CAD build for the part. Positions are in the model's coordinates, mm. A direction names the side the tool comes from. Give positions to 0.01 mm unless a question says otherwise; leave off trailing zeros. Write each loop counter-clockwise with the first axis right and the second up, starting at its lowest first coordinate (ties: lowest second). Pieces come first, ordered by that corner, then holes. Notation, with made-up numbers: (13.25, -35.5) - (22.25, -35.5) arc R18 cw to (22.25, -26.5) - close; hole circle Ø6 at (58.25, 39). An arc over 180 degrees is marked (long way). Put each result on its own line as item: value. Start each with the question number.
1. Tool access for faces 1 (the flat face through (-3, -47.498, 12.2)), 2 (the flat face through (0, -60.198, 7)): list every direction of +Z, -Z, +X, -X, +Y, -Y with a clear straight run to the whole face (end or side of a thin tool).
2. Cut at C-C on y = -6. List the corners of the cut face in (x, z).
3. Cut at D-D on y = -49.5. List the corners of the cut face in (x, z), and give its area (3 significant figures).
4. Cut at B-B on z = 6.35. List the corners of the cut face in (x, y).
5. Wall check: line 1 (X direction, y = -53, z = 7); line 2 (Y direction, x = -1.25, z = -0.75); line 3 (Z direction, x = 0.25, y = -42). Give the ranges that are in metal, low to high.
6. Cut at A-A on x = 0. List the corners of the cut face in (y, z).
7. Drop flat-ended pins along their axis: pin 1 (2 mm diameter, centred on x = 9, y = -8.5, fed in from +Z); pin 2 (3 mm diameter, centred on x = -6.5, y = 35.5, fed in from -Z); pin 3 (12 mm diameter, centred on x = 8, y = -43, fed in from +Z); pin 4 (12 mm diameter, centred on y = -32.5, z = 0, fed in from -X). Give the stop position or say it passes through.
from build123d import *

# Parameters (mm, degrees)
F0_R       = 6.35
F1_DEPTH   = 101.6
F1_FACE1_R = 6.35
F2_R       = 12.7
F2_R_2     = 6.35
F1_FACE_R  = 6.35
F3_DEPTH   = 6.35


with BuildPart() as f1:
    # F0 (on Front) → F1 (new body)
    with BuildSketch(Plane.XZ):
        with Locations((0, 6.35)):
            Circle(F0_R)
    extrude(amount=F1_DEPTH)

    # F1_face1 (on face) + F2 (on face) + F1_face (on face) → F3 (join, symmetric)
    with BuildSketch(Plane(origin=(0, 0, 6.35), x_dir=(1, 0, 0), z_dir=(0, 1, 0))):
        Circle(F1_FACE1_R)
    with BuildSketch(Plane.XZ.offset(101.6)):
        with Locations((0, 6.35)):
            Circle(F2_R)
        with Locations((0, 6.35)):
            Circle(F2_R_2, mode=Mode.SUBTRACT)
        with Locations((0, 6.35)):
            Circle(F2_R_2)
    with BuildSketch(Plane(origin=(0, -101.6, 6.35), x_dir=(1, 0, 0), z_dir=(0, -1, 0))):
        Circle(F1_FACE_R)
    extrude(amount=F3_DEPTH, both=True, dir=(0, 1, 0))


with BuildPart() as f1_1:
    # F4: moved
    add(f1.part.moved(Location((0, 47.752, 0))))


solid = f1_1.part
Report:
1. face 1: +Y
1. face 2: +Z, -Z, +X, -X, -Y
2. outline: circle Ø12.7 at (0, 6.35)
3. outline: circle Ø25.4 at (0, 6.35)
3. area: 507 mm²
4. outline: (-12.7, -60.2) - (12.7, -60.2) - (12.7, -47.5) - (6.35, -47.5) - (6.35, 54.1) - (-6.35, 54.1) - (-6.35, -47.5) - (-12.7, -47.5) - close
5. line 1: x = -12.68 to 12.68
5. line 2: y = -60.2 to -47.5
5. line 3: z = 0 to 12.7
6. outline: (-60.2, -6.35) - (-47.5, -6.35) - (-47.5, 0) - (54.1, 0) - (54.1, 12.7) - (-47.5, 12.7) - (-47.5, 19.05) - (-60.2, 19.05) - close
7. pin 1: passes through
7. pin 2: stops at z = 2.44
7. pin 3: stops at z = 18.39
7. pin 4: stops at x = -6.34
